Verification items for the finished model (mm, model axes). Face numbers are marked on the shaded views. A direction names the side the tool comes from. Give positions to 0.01 mm unless a question says otherwise; leave off trailing zeros. Loops run counter-clockwise (first coordinate to the right, second up) from the corner with the lowest first, then second, coordinate; pieces in that order, holes last. Notation, with made-up numbers: M 64,22 L 87,22 A20 ccw 87,52 Z; hole C 57.5,58 d2. An arc over 180 degrees is marked long. Use a Markdown table: item, result.
Autodesk Inventor part; units mm, degrees
ref_plane "YZ Plane" through (0, 0, 0) normal (1, 0, 0) x (0, 1, 0)
ref_plane "XZ Plane" through (0, 0, 0) normal (0, 1, 0) x (-1, 0, 0)
ref_plane "XY Plane" through (0, 0, 0) normal (0, 0, 1) x (1, 0, 0)
sketch "草图1" plane through (0, 0, 0) normal (0, 0, 1) x (1, 0, 0)
  circle A0 centre (0, 0) radius 6
  dimension "d0" = 12
extrude "拉伸1" add sketch "草图1" along normal blind 1.5
sketch "草图2" plane through (0, 0, 1.5) normal (0, 0, 1) x (1, 0, 0)
  line L0 (0, -4.6188) -> (-4, -2.3094)
  line L1 (-4, -2.3094) -> (-4, 2.3094)
  line L2 (-4, 2.3094) -> (0, 4.6188)
  line L3 (0, 4.6188) -> (4, 2.3094)
  line L4 (4, 2.3094) -> (4, -2.3094)
  line L5 (4, -2.3094) -> (0, -4.6188)
  line L6 (0, 0) -> (0, 2.9591)
  dimension "d3" = 8
  dimension "d4" = 2.9591
extrude "拉伸2" add sketch "草图2" along normal blind 5
sketch "草图3" plane through (0, 0, 0) normal (0, 0, -1) x (-1, 0, 0)
  circle A0 centre (0, 0) radius 4
  dimension "d7" = 8
extrude "拉伸3" add sketch "草图3" along normal blind 28
thread "螺纹1"
chamfer "倒角1" distance 0.5 angle 45 1 edges at (4, 0, -28)
fillet "圆角1" radius 0.5 13 edges at (-6, 0, 1.5) (4, 0, 6.5) (2, 3.4641, 6.5) (-2, 3.4641, 6.5) (-4, 0, 6.5) (-2, -3.4641, 6.5) (2, -3.4641, 6.5) (4, 2.3094, 4) (0, 4.6188, 4) (4, -2.3094, 4) (0, -4.6188, 4) (-4, -2.3094, 4) (-4, 2.3094, 4)
properties part number "装填斗固定螺丝"
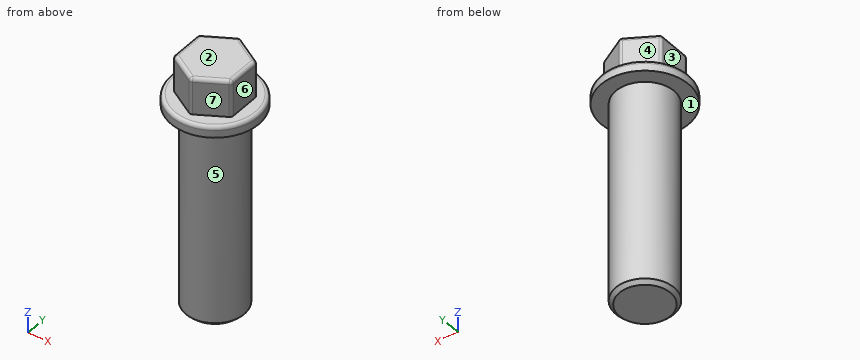
(1) Cross-section at A-A on y = 0. Record the cut outline in (x, z), then the cut area to 3 significant figures.
Results below:
| item | result |
|---|---|
| outline | M -6,0 L -4,0 L -4,-27.5 L -3.5,-28 L 3.5,-28 L 4,-27.5 L 4,0 L 6,0 L 6,1 A0.5 ccw 5.5,1.5 L 4,1.5 L 4,6 A0.5 ccw 3.5,6.5 L -3.5,6.5 A0.5 ccw -4,6 L -4,1.5 L -5.5,1.5 A0.5 ccw -6,1 Z |
| area | 282 mm^2 |
(2) Material ranges on line 1 (Z direction, x = -5, y = 2.25); line 2 (Y direction, x = 1, z = -7); line 3 (X direction, y = -3.5, z = -16), recorded low to high.
Results below:
| item | result |
|---|---|
| line 1 | 0 to 1.5 |
| line 2 | -3.87 to 3.87 |
| line 3 | -1.94 to 1.94 |
(3) Draft check along Y on the marked faces 4, 5, 6 and 7. Enter one of: +Y half, -Y half, draft (parallel to the pull), parting line (faces both ways), or undercut.
Results below:
| item | result |
|---|---|
| face 4 | +Y half |
| face 5 | parting line |
| face 6 | draft |
| face 7 | -Y half |
(4) Cross-section at B-B on z = -10. Record the cut outline in (x, y), then the cut area to 3 significant figures.
Results below:
| item | result |
|---|---|
| outline | C 0,0 d8 |
| area | 50.3 mm^2 |
(5) Gauge pin test, flat ends, axial feed: P1, Ø5, axis at x = 1, z = -16.5, coming from the +Y side; P2, Ø1.2, axis at y = 0.5, z = 4, coming from the -X side; P3, Ø2, axis at x = -3.5, z = -4, coming from the -Y side. Record the tip position at first contact, or that the pin passes through.
Results below:
| item | result |
|---|---|
| P1 | y = 4 |
| P2 | x = -4 |
| P3 | y = -3.12 |
(6) Set-up check for the marked faces 1, 2 and 3: record each of +Z, -Z, +X, -X, +Y, -Y from which the full face is reachable in a straight line by a thin tool's end or side.
Results below:
| item | result |
|---|---|
| face 1 | -Z |
| face 2 | +Z, +X, -X, +Y, -Y |
| face 3 | +Z, -X, +Y, -Y |
